Input: part model. Units: mm. Frame: model coordinates. Face numbers are marked on the shaded views. A direction names the side the tool comes from. Give positions to 0.01 mm unless a question says otherwise; leave off trailing zeros. Loops run counter-clockwise (first coordinate to the right, second up) from the corner with the lowest first, then second, coordinate; pieces in that order, holes last. Notation, with made-up numbers: (71.5, 69) - (85.5, 69) arc R15 cw to (85.5, 81) - close; hole circle Ø1 at (55, -36.5). An arc over 180 degrees is marked (long way). Answer as a JSON object with one key per item and string values. Group by question number.
(1) Material intervals for L1, parallel to X at y = 5.5, z = 1.25; L2, parallel to Z at x = 35, y = 1.1, sorted ascending.
(2) Section query C-C (z = -35). Return loops of the section in (x, y).
(3) Section query B-B (y = 5.5). Return loops of the section in (x, z).
(4) Access query for the marked faces 1, 2 and 3. Directions: +Z, -Z, +X, -X, +Y, -Y. A direction counts if a zero-diameter tool reaches every point of the face in a straight line with its end or side. Return the directions, or none.
(5) Section query A-A (x = -21). Return loops of the section in (y, z).
(6) Pin query (flat end, axial travel): P1, Ø4, axis at x = -35, z = -35, coming from the +Y side; P2, Ø1.8, axis at x = -35, z = 35, coming from the +Y side; P3, Ø2.5, axis at x = 37, y = 4, coming from the -Z side. Return the tip coordinate at first contact, or that it passes through.
(7) Section query D-D (z = 4). Return loops of the section in (x, y).
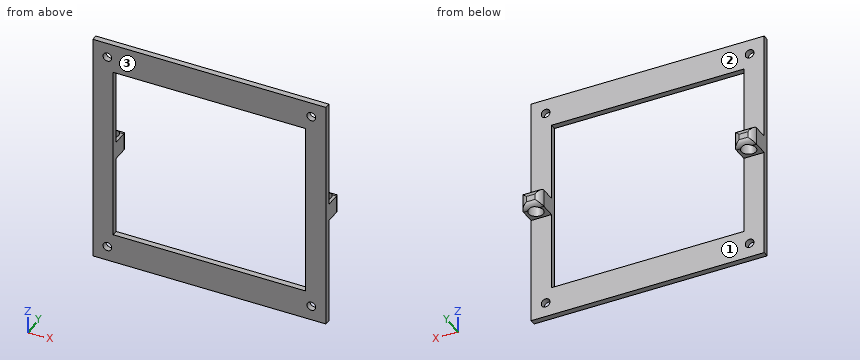
Autodesk Inventor part; units mm, degrees
ref_plane "YZ Plane" through (0, 0, 0) normal (1, 0, 0) x (0, 1, 0)
ref_plane "XZ Plane" through (0, 0, 0) normal (0, 1, 0) x (-1, 0, 0)
ref_plane "XY Plane" through (0, 0, 0) normal (0, 0, 1) x (1, 0, 0)
sketch "Esquisse1" plane through (0, 0, 0) normal (0, 1, 0) x (-1, 0, 0)
  line L0 (-40, 40) -> (40, 40)
  line L1 (40, 40) -> (40, -40)
  line L2 (40, -40) -> (-40, -40)
  line L3 (-40, -40) -> (-40, 40)
  line L4 (-40, 40) -> (40, -40) construction
  line L5 (40, 40) -> (-40, -40) construction
  point P0 (0, 0)
  dimension "d0" = 80
extrude "Extrusion1" add sketch "Esquisse1" along normal blind 2
sketch "Esquisse2" plane through (0, 2, 0) normal (0, 1, 0) x (1, 0, 0)
  point P0 (0, 0)
sketch "Esquisse3" plane through (0, 2, 0) normal (0, 1, 0) x (1, 0, 0)
  line L0 (33, -30) -> (-33, -30)
  line L1 (-33, -30) -> (-33, 30)
  line L2 (-33, 30) -> (33, 30)
  line L3 (33, 30) -> (33, -30)
  line L4 (33, -30) -> (-33, 30) construction
  line L5 (-33, -30) -> (33, 30) construction
  point P0 (0, 0)
  dimension "d3" = 66
  dimension "d4" = 60
extrude "Extrusion2" cut sketch "Esquisse3" against normal blind 10
sketch "Esquisse10" plane through (0, 2, 0) normal (0, 1, 0) x (1, 0, 0)
  line L0 (35, 35) -> (-35, 35)
  line L1 (-35, 35) -> (-35, -35)
  line L2 (-35, -35) -> (35, -35)
  line L3 (35, -35) -> (35, 35)
  line L4 (35, 35) -> (-35, -35) construction
  line L5 (-35, 35) -> (35, -35) construction
  line L6 (-40, 40) -> (-40, -40)
  line L7 (-40, -40) -> (40, -40)
  point P0 (0, 0)
  point P1 (-40, -5)
  dimension "d23" = 5
  dimension "d24" = 5
hole "Perçage1" at (35, 2, 35) at (-35, 2, 35) at (-35, 2, -35) at (35, 2, -35) direction (0, -1, 0) diameter 3 depth 66.675 tip angle 118
sketch "Esquisse11" plane through (0, 2, 0) normal (0, 1, 0) x (1, 0, 0)
  line L0 (40, -40) -> (40, 40)
  line L1 (33, 30) -> (33, -30)
  line L2 (40, 3) -> (33, 3)
  line L3 (33, 3) -> (33, -3)
  line L4 (33, -3) -> (40, -3)
  line L5 (40, -3) -> (40, 3)
  point P0 (0, 0)
  dimension "d37" = 3
  dimension "d38" = 3
extrude "Extrusion9" add sketch "Esquisse11" along normal blind 7
sketch "Esquisse12" plane through (40, 2, -3) normal (0, 0, -1) x (-1, 0, 0)
  line L0 (7, 0) -> (0, 0)
  line L1 (0, 0) -> (7, 6.8816)
  line L2 (0, 0) -> (0, 7)
  line L3 (7, 0) -> (0, 7)
  point P0 (40, -2)
  point P1 (3.5, 3.5)
hole "Perçage2" at (36.5, 5.5, -3) direction (0, 0, 1) diameter 5 depth 66.675 tip angle 118
fillet "Congé1" radius 2 4 edges at (36.5, 9, -3) (40, 9, 0) (36.5, 9, 3) (33, 9, 0)
ref_plane "Plan de construction1" through (0, 0, -40) normal (-1, 0, 0) x (0, 0, 1)
mirror "Symétrie1" about plane through (0, 0, -40) normal (-1, 0, 0) of "Extrusion9", "Perçage2", "Congé1"
Recorded:
{
 "1": {"L1": "x = -40 to -39, -34 to -33, 33 to 34, 39 to 40", "L2": "z = -40 to -36.5, -33.5 to 33.5, 36.5 to 40"},
 "2": {"outline": "(-40, 0) - (-36.5, 0) - (-36.5, 2) - (-40, 2) - close; (-33.5, 0) - (33.5, 0) - (33.5, 2) - (-33.5, 2) - close; (36.5, 0) - (40, 0) - (40, 2) - (36.5, 2) - close"},
 "3": {"outline": "(-40, -3) - (-39, -3) - (-39, 3) - (-40, 3) - close; (-34, -3) - (-33, -3) - (-33, 3) - (-34, 3) - close; (33, -3) - (34, -3) - (34, 3) - (33, 3) - close; (39, -3) - (40, -3) - (40, 3) - (39, 3) - close"},
 "4": {"face 1": "-Z, +X, -X, +Y", "face 2": "+Z, +X, -X, +Y", "face 3": "+Z, -Z, +X, -X, -Y"},
 "5": {"outline": "(0, -40) - (2, -40) - (2, -30) - (0, -30) - close; (0, 30) - (2, 30) - (2, 40) - (0, 40) - close"},
 "6": {"P1": "stops at y = 2", "P2": "passes through", "P3": "stops at z = -3"},
 "7": {"outline": "(-40, 0) - (-33, 0) - (-33, 2) - (-40, 2) - close; (33, 0) - (40, 0) - (40, 2) - (33, 2) - close"}
}
